Input: part model. Units: mm. Frame: model coordinates. Round coordinates to 2 decimals unless told otherwise and drop trailing zeros. Write each loop counter-clockwise with the first axis right and the second up, starting at its lowest first coordinate (ties: lowest second). Pieces come first, ordered by that corner, then holes. Notation, with made-up numbers: M -13,-8 L 12,-8 A29 ccw 12,13 Z; hole C -21,-16 d6. An arc over 180 degrees is marked long. Answer as CSV lines item,"result". Start each with the question number.
```python
from build123d import *

# Parameters (mm, degrees)
F0_R     = 12.5
F1_DEPTH = 3


with BuildPart() as f1:
    # F0 (on Top) → F1 (new body)
    with BuildSketch(Plane.XY):
        with BuildLine():
            Line((-17.870255, 414.621119), (2.345661, 474.068432))
            ThreePointArc((2.345661, 474.068432), (-377.797369, 190.367681), (-166.401004, -234.257349))
            Line((-166.401004, -234.257349), (-17.870255, 3.655279))
            Line((-17.870255, 3.655279), (-17.870255, 104.621119))
            Line((-17.870255, 104.621119), (-17.870255, 414.621119))
        make_face()
        with Locations((-187.870255, 272.119941)):
            Circle(F0_R, mode=Mode.SUBTRACT)
    extrude(amount=F1_DEPTH)


solid = f1.part
```
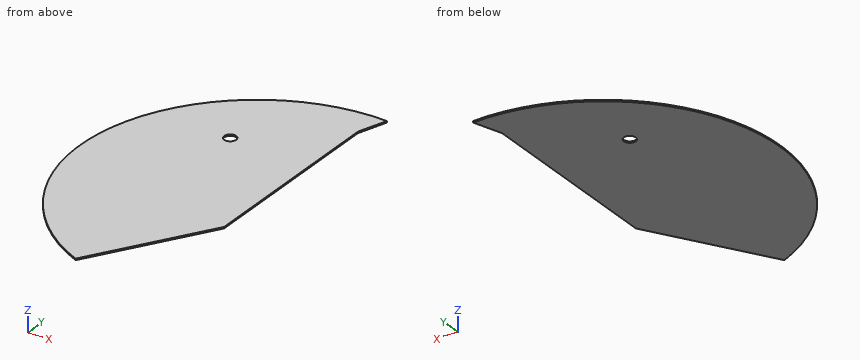
Item 1: Cut plane C-C, the plane x = -113. Return loops of the section in (y, z), plus the area to 3 significant figures.
Item 2: Line query: line 1 (X direction, y = 113, z = 2.25); line 2 (X direction, y = 278, z = 2.7); line 3 (X direction, y = 279.5, z = 2.7). Output: solid intervals per line, ascending. Write a range as [from, to].
Item 3: Cut plane A-A, the plane z = 1.1. Return loops of the section in (x, y).
Item 4: Cut plane B-B, the plane y = 50. Return loops of the section in (x, z).
Item 5: Pin query (flat end, axial travel): pin 1 Ø1 at (x, z) = (-250, 1) entering from -Y; pin 2 Ø1.5 at (x, y) = (-208, -111.5) entering from -Z. Return the tip coordinate at first contact, or that it passes through.
Results list:
1,outline,"M -148.72,0 L 462.18,0 L 462.18,3 L -148.72,3 Z"
1,area,"1,830 mm²"
2,line 1,"[-387.78, -17.87]"
2,line 2,"[-344.73, -198.9], [-176.84, -17.87]"
2,line 3,"[-343.93, -197.96], [-177.78, -17.87]"
3,outline,"M -166.4,-234.26 L -17.87,3.66 L -17.87,414.62 L 2.35,474.07 A370 ccw Z; hole C -187.87,272.12 d25"
4,outline,"M -383.82,0 L -17.87,0 L -17.87,3 L -383.82,3 Z"
5,pin 1,"y = -183.91"
5,pin 2,"z = 0"
